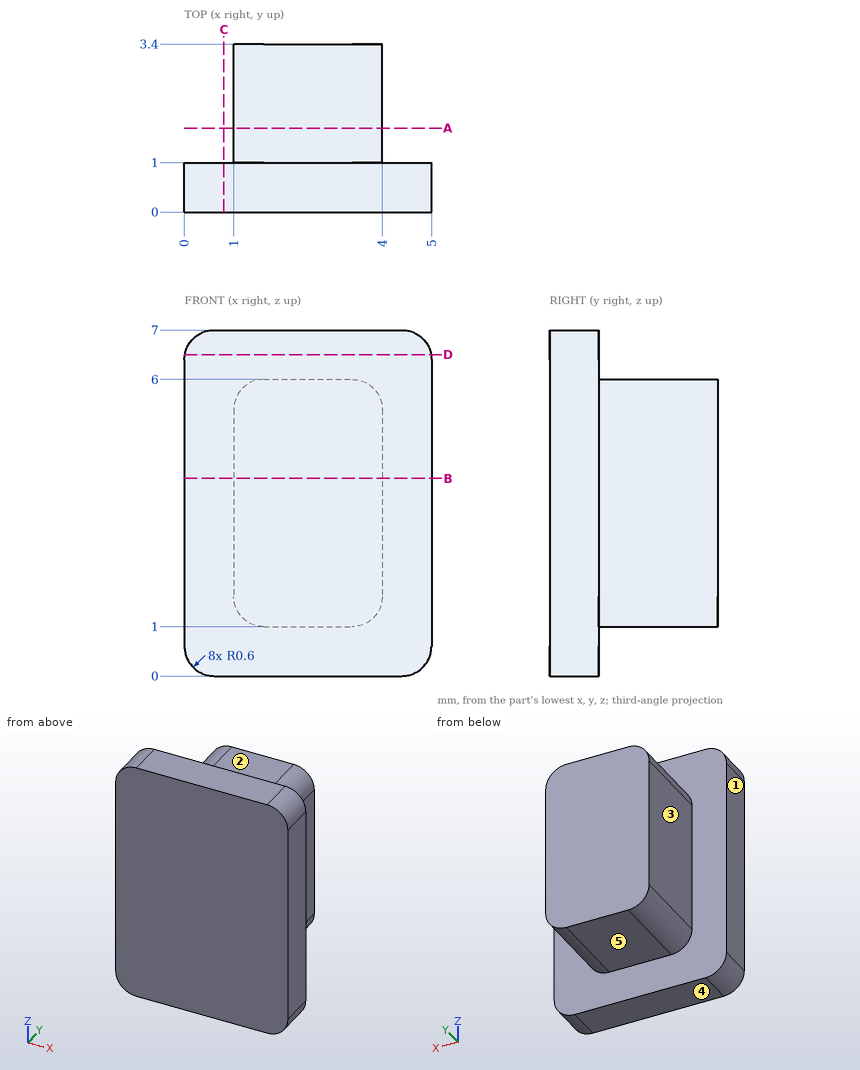
For this review, use the dimensioned drawing (mm, ordinates from the lowest corner) and the shaded views. A direction names the side the tool comes from. Coordinates: 2 decimals unless noted, no trailing zeros. Order: outer loops, then holes, each group sorted by start corner. A loop starts at its lowest first (then second) coordinate and runs counter-clockwise, first axis right, second up. Notation, with made-up numbers: (35, 11) -> (65, 11) arc R33 ccw to (65, 40) -> close; hole circle Ø5 at (65, -23.5). An arc over 180 degrees is marked (long way). One line per item, written item: value. Start each with the question number.
Q1. Take a section at B-B, the plane z = 4. State the section outline as (x, y) points.
Q2. Take a section at A-A, the plane y = 1.7. State the section outline as (x, z) points, then the cut area to 3 significant figures.
Q3. Take a section at D-D, the plane z = 6.5. State the section outline as (x, y) points.
Q4. Take a section at C-C, the plane x = 0.8. State the section outline as (y, z) points, then the cut area to 3 significant figures.
Q5. Insertion check: pin 1 Ø1.4 at (x, y) = (2.5, 3) entering from +Z; pin 2 Ø0.5 at (x, y) = (2, 2.5) entering from -Z; pin 3 Ø0.7 at (y, z) = (2, 3) entering from +X. Each pin has a flat end and moves straight along its axis. Give the tip position at first contact, or say it passes through.
Q6. For probe 1 along Z at (x, y) = (2.15, 2.4); probe 2 along Y at (x, z) = (4.6, 5.5); probe 3 along X at (y, z) = (2.3, 3), list the stretches that pass through material, from the lowest coordinate up.
Q7. Tool access review of the marked faces 1, 2, 3, 4 and 5: name each direction out of +Z, -Z, +X, -X, +Y, -Y from which nothing blocks a thin tool from reaching the whole face with its end or side.
Values follow:
1. outline: (0, 0) -> (5, 0) -> (5, 1) -> (4, 1) -> (4, 3.4) -> (1, 3.4) -> (1, 1) -> (0, 1) -> close
2. outline: (1, 1.6) arc R0.6 ccw to (1.6, 1) -> (3.4, 1) arc R0.6 ccw to (4, 1.6) -> (4, 5.4) arc R0.6 ccw to (3.4, 6) -> (1.6, 6) arc R0.6 ccw to (1, 5.4) -> close
2. area: 14.7 mm2
3. outline: (0.01, 0) -> (4.99, 0) -> (4.99, 1) -> (0.01, 1) -> close
4. outline: (0, 0) -> (1, 0) -> (1, 7) -> (0, 7) -> close
4. area: 7.00 mm2
5. pin 1: stops at z = 6
5. pin 2: stops at z = 1
5. pin 3: stops at x = 4
6. probe 1: z = 1 to 6
6. probe 2: y = 0 to 1
6. probe 3: x = 1 to 4
7. face 1: +Z, -Z, -X, +Y, -Y
7. face 2: +Z, +X, -X, +Y
7. face 3: +Z, -Z, -X, +Y
7. face 4: -Z, +X, -X, +Y, -Y
7. face 5: -Z, +X, -X, +Y
